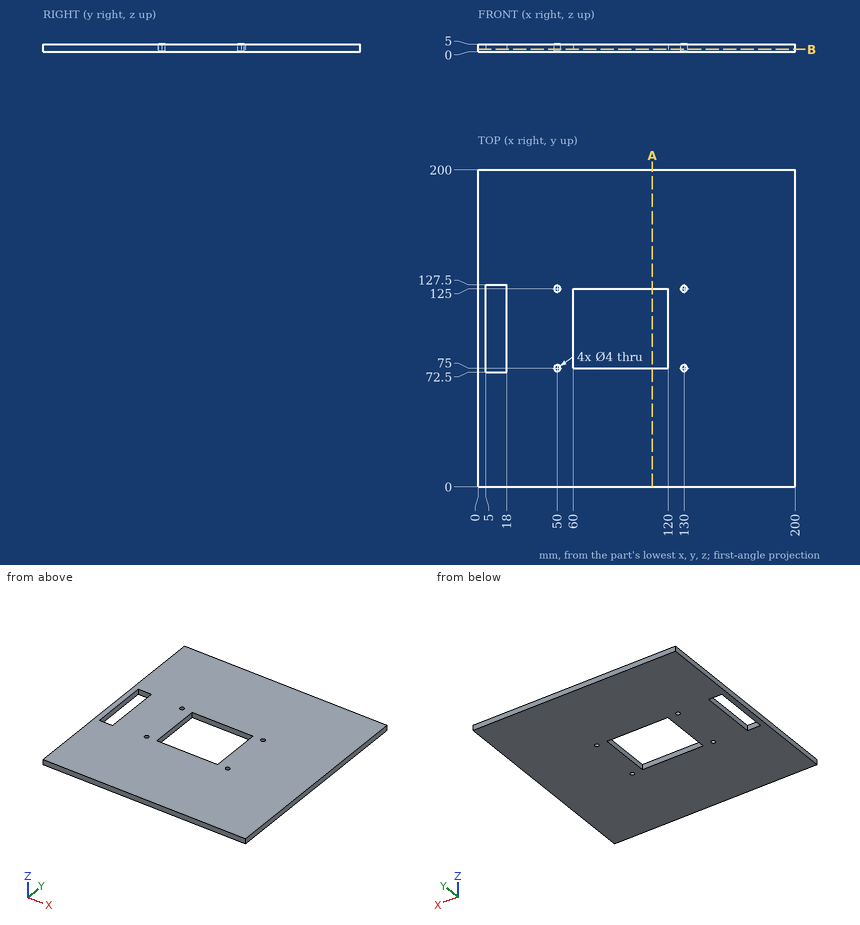
Geometry check sheet. Reference: drawing and pictorial views, mm from the part's lowest x, y, z. Round coordinates to 2 decimals unless told otherwise and drop trailing zeros. Loops run counter-clockwise (first coordinate to the right, second up) from the corner with the lowest first, then second, coordinate; pieces in that order, holes last. Notation, with made-up numbers: (40.5, 75.5) -> (67.5, 75.5) arc R6 cw to (67.5, 85.5) -> close; hole circle Ø10 at (71.5, 35.5). An arc over 180 degrees is marked (long way). Use a Markdown table: item, result.
(1) Sectioned sample at B-B (z = 1.6). Enter the section's corners in (x, y), then the cut area to 3 significant figures.
Calculated:
| item | result |
|---|---|
| outline | (0, 0) -> (200, 0) -> (200, 200) -> (0, 200) -> close; hole (5, 72.5) -> (18, 72.5) -> (18, 127.5) -> (5, 127.5) -> close; hole circle Ø4 at (50, 75); hole circle Ø4 at (50, 125); hole (60, 75) -> (120, 75) -> (120, 125) -> (60, 125) -> close; hole circle Ø4 at (130, 75); hole circle Ø4 at (130, 125) |
| area | 36,200 mm² |
(2) Go/stop test with a flat-tipped pin: P1, Ø6.5, axis at x = 50, y = 125, coming from the +Z side. Record where the tip stops, or that it passes through.
Calculated:
| item | result |
|---|---|
| P1 | z = 5 |
(3) Scan lines: probe 1 along X at (y, z) = (91.5, 3); probe 2 along Y at (x, z) = (130, 2.6); probe 3 along Y at (x, z) = (49, 3.5). Record each from-to range of solid material in increasing order.
Calculated:
| item | result |
|---|---|
| probe 1 | 0 to 5, 18 to 60, 120 to 200 |
| probe 2 | 0 to 73, 77 to 123, 127 to 200 |
| probe 3 | 0 to 73.27, 76.73 to 123.27, 126.73 to 200 |
(4) Sectioned sample at A-A (x = 110). Enter the section's corners in (y, z).
Calculated:
| item | result |
|---|---|
| outline | (0, 0) -> (75, 0) -> (75, 5) -> (0, 5) -> close; (125, 0) -> (200, 0) -> (200, 5) -> (125, 5) -> close |
